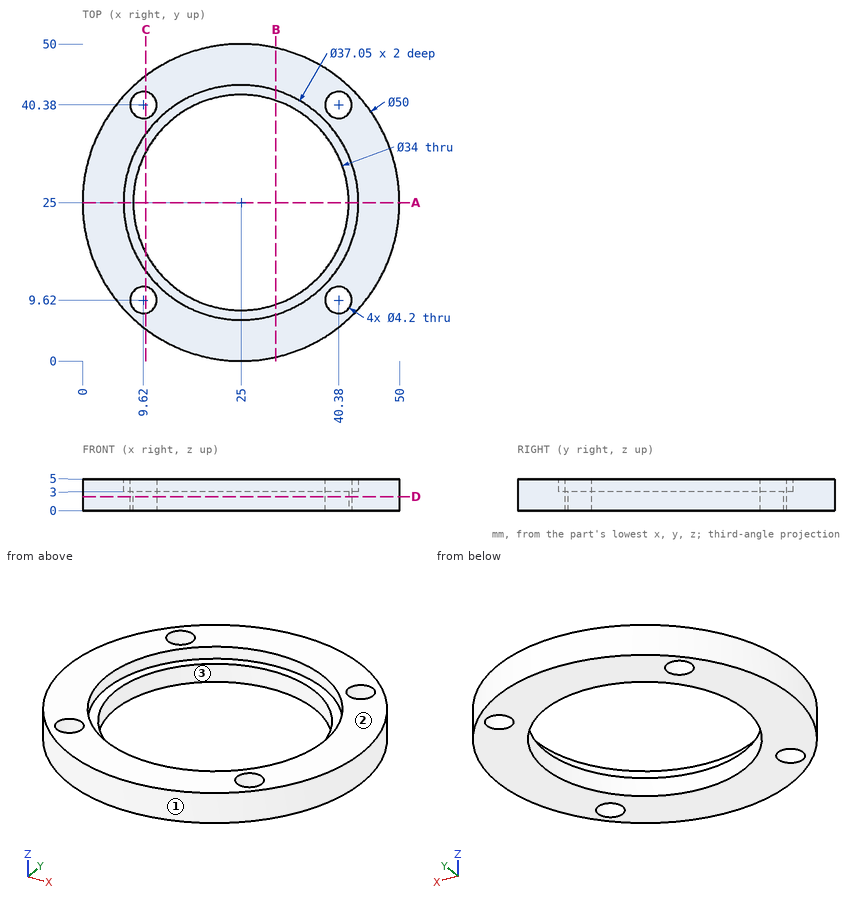
Design review of the part shown in the three views and the two pictorial views. Dimensions are in mm from the part's minimum x, y and z. Coordinates: 2 decimals unless noted, no trailing zeros. Loops run counter-clockwise (first coordinate to the right, second up) from the corner with the lowest first, then second, coordinate; pieces in that order, holes last.
(1) Consider section D-D, the plane z = 2.2. Give the boundary of the cut face in (x, y), plus the area to 3 significant figures.
Determined:
outline: circle Ø50 at (25, 25); hole circle Ø4.2 at (9.62, 9.62); hole circle Ø4.2 at (9.62, 40.38); hole circle Ø34 at (25, 25); hole circle Ø4.2 at (40.38, 9.62); hole circle Ø4.2 at (40.38, 40.38)
area: 1,000 mm2
(2) Consider section A-A, the plane y = 25. Give the boundary of the cut face in (x, z) (1 decimal), plus the area to 3 significant figures.
Determined:
outline: (0, 0) - (8, 0) - (8, 3) - (6.5, 3) - (6.5, 5) - (0, 5) - close; (42, 0) - (50, 0) - (50, 5) - (43.5, 5) - (43.5, 3) - (42, 3) - close
area: 73.9 mm2
(3) Draft analysis for pull direction X (two halves, no side actions). For the marked faces 1, 2 and 3, state which applies: +X half, -X half, draft (parallel to the pull), parting line (faces both ways), or undercut.
Determined:
face 1: parting line
face 2: draft
face 3: undercut
(4) Consider section C-C, the plane x = 10. Give the boundary of the cut face in (y, z) (1 decimal).
Determined:
outline: (5, 0) - (7.6, 0) - (7.6, 5) - (5, 5) - close; (11.7, 0) - (17, 0) - (17, 3) - (14.1, 3) - (14.1, 5) - (11.7, 5) - close; (33, 0) - (38.3, 0) - (38.3, 5) - (35.9, 5) - (35.9, 3) - (33, 3) - close; (42.4, 0) - (45, 0) - (45, 5) - (42.4, 5) - close
(5) Insertion check: P1, Ø1.5, axis at y = 44.5, z = 3, coming from the +X side (1 decimal); P2, Ø1.5, axis at y = 39.5, z = 4, coming from the -X side; P3, Ø2.5, axis at x = 40.38, y = 9.62, coming from the -Z side. Each pin has a flat end and moves straight along its axis. Give the tip position at first contact, or say it passes through.
Determined:
P1: stops at x = 41.5
P2: stops at x = 4.12
P3: passes through
(6) Consider section B-B, the plane x = 30.5. Give the boundary of the cut face in (y, z) (1 decimal).
Determined:
outline: (0.6, 0) - (8.9, 0) - (8.9, 3) - (7.3, 3) - (7.3, 5) - (0.6, 5) - close; (41.1, 0) - (49.4, 0) - (49.4, 5) - (42.7, 5) - (42.7, 3) - (41.1, 3) - close
(7) Wall thickness on L1, parallel to Y at x = 12, z = 0.4 (1 decimal); L2, parallel to Y at x = 24, z = 0.3; L3, parallel to Z at x = 32, y = 42: over which ranges is each line inside the solid? List them lowest first.
Determined:
L1: y = 3.6 to 14, 36 to 46.4
L2: y = 0.02 to 8.03, 41.97 to 49.98
L3: z = 0 to 3
